```python
from build123d import *

# Parameters (mm, degrees)
SKETCH_1_W          = 88
SKETCH_1_H          = 60.2
EXTRUDE_1_DEPTH     = 16
SKETCH_1_4_R        = 5
SKETCH_1_4_R_2      = 9.5
EXTRUDE_3_DEPTH     = 23
SKETCH_2_R          = 4
EXTRUDE_4_DEPTH     = 30
CUT_EXTRUDE_3_DEPTH = 15
SKETCH_4_R          = 1.5
CUT_EXTRUDE_4_DEPTH = 10
EXTRUDE_6_DEPTH     = 16
EXTRUDE_7_DEPTH     = 2
SKETCH_7_R          = 22.25
EXTRUDE_8_DEPTH     = 66.5


with BuildPart() as part:
    # 草图1 → 凸台-拉伸1 (new body)
    with BuildSketch(Plane(origin=(0, 0, 0), x_dir=(1, 0, 0), z_dir=(0, 1, 0))):
        Rectangle(SKETCH_1_W, SKETCH_1_H)
    extrude(amount=EXTRUDE_1_DEPTH)

    # 草图1<4> → 凸台-拉伸3 (add)
    with BuildSketch(Plane(origin=(0, 0, 0), x_dir=(1, 0, 0), z_dir=(0, 1, 0))):
        with Locations((-20.4, 20)):
            Circle(SKETCH_1_4_R)
        with Locations((19.6, 20)):
            Circle(SKETCH_1_4_R)
        with Locations((19.6, -20)):
            Circle(SKETCH_1_4_R)
        with Locations((-20.4, -20)):
            Circle(SKETCH_1_4_R)
        with Locations((-20.4, 0)):
            Circle(SKETCH_1_4_R_2)
    extrude(amount=EXTRUDE_3_DEPTH)

    # 草图2 → 凸台-拉伸4 (add)
    with BuildSketch(Plane(origin=(0, 23, 0), x_dir=(1, 0, 0), z_dir=(0, 1, 0))):
        with Locations((-20.4, 0)):
            Circle(SKETCH_2_R)
    extrude(amount=EXTRUDE_4_DEPTH)

    # 草图3 → 切除-拉伸3 (cut)
    with BuildSketch(Plane(origin=(0, 53, 0), x_dir=(1, 0, 0), z_dir=(0, 1, 0))):
        with BuildLine():
            Line((-23.864101615, 2), (-16.935898385, 2))
            ThreePointArc((-16.935898385, 2), (-20.4, 4), (-23.864101615, 2))
        make_face()
    extrude(amount=-CUT_EXTRUDE_3_DEPTH, mode=Mode.SUBTRACT)

    # 草图4 → 切除-拉伸4 (cut)
    with BuildSketch(Plane(origin=(0, 23, 0), x_dir=(1, 0, 0), z_dir=(0, 1, 0))):
        with Locations((-20.4, 20)):
            Circle(SKETCH_4_R)
        with Locations((19.6, 20)):
            Circle(SKETCH_4_R)
        with Locations((19.6, -20)):
            Circle(SKETCH_4_R)
        with Locations((-20.4, -20)):
            Circle(SKETCH_4_R)
    extrude(amount=-CUT_EXTRUDE_4_DEPTH, mode=Mode.SUBTRACT)

    # 草图5 → 凸台-拉伸6 (add)
    with BuildSketch(Plane(origin=(0, 0, 0), x_dir=(1, 0, 0), z_dir=(0, 1, 0))):
        with BuildLine():
            Line((44, -30.1), (44, 30.1))
            ThreePointArc((44, 30.1), (50.801977879, 0), (44, -30.1))
        make_face()
    extrude(amount=EXTRUDE_6_DEPTH)

    # 草图6 → 凸台-拉伸7 (add)
    with BuildSketch(Plane.XZ):
        with BuildLine():
            Line((18, -16), (48.948878029, -16))
            ThreePointArc((48.948878029, -16), (50.801977879, 0), (48.948878029, 16))
            Line((48.948878029, 16), (18, 16))
            Line((18, 16), (18, -16))
        make_face()
    extrude(amount=EXTRUDE_7_DEPTH)

    # 草图7 → 凸台-拉伸8 (add)
    with BuildSketch(Plane.XZ.offset(2)):
        with Locations((34.40098894, 0)):
            Circle(SKETCH_7_R)
    extrude(amount=EXTRUDE_8_DEPTH)


solid = part.part
```
Could you check a few things on this model? Use its own coordinates, in mm. A direction names the side the tool comes from. Give positions to 0.01 mm unless a question says otherwise; leave off trailing zeros. Order: outer loops, then holes, each group sorted by start corner. A loop starts at its lowest first (then second) coordinate and runs counter-clockwise, first axis right, second up.
Q1. If I drill on line 1 along X through (y, z) = (21, -20); line 2 along Z through (x, y) = (19.6, 19); line 3 along Z through (x, y) = (19, 15), over which ranges is the centre line in solid material (lowest first)?
Q2. Suppose I cut it at B-B, the plane z = 20. Write out the boundary of the cut face in (x, y), and give its area (3 significant figures).
Q3. We'd pull the mould along Z, two halves only. Please class faces 1 (the flat face through (34, -68.5, 0)), 2 (the cylindrical face through (18.1, 18.07, 19.93)), 3 (the flat face through (-1, 8, 30.1)): +Z half, -Z half, draft (parallel to the pull), parting line (faces both ways), or undercut.
Q4. Suppose I cut it at A-A, the plane z = 0. Write out the boundary of the cut face in (x, y), and give its area (3 significant figures).
Q5. I'm going to push flat-ended pins straight in: P1, Ø1, axis at x = -21, z = -3, coming from the +Y side; P2, Ø2, axis at y = -6, z = -15.5, coming from the +X side; P3, Ø11, axis at x = 19, z = -22, coming from the +Y side; P4, Ø9.5, axis at x = -21.5, z = -4.5, coming from the +Y side. Where does each tip first touch, or does it pass through?
Q6. For faces 4 (the flat face through (-22, 23, 21)), 5 (the flat face through (-20, 46, -2)), 6 (the flat face through (-16, 23, 0)), which set-ups out of +Z, -Z, +X, -X, +Y, -Y let a thin tool reach every point of the face, with its end or its side?
Q7. Suppose I cut it at D-D, the plane y = 41. Write out the boundary of the cut face in (x, z).
Solution:
1. line 1: x = -25.4 to -21.9, -18.9 to -15.4, 14.6 to 18.1, 21.1 to 24.6
1. line 2: z = -25 to -21.5, -18.5 to -15, 15 to 18.5, 21.5 to 25
1. line 3: z = -30.1 to -21.37, -18.63 to 18.63, 21.37 to 30.1
2. outline: (-44, 0) - (47.88, 0) - (47.88, 16) - (24.6, 16) - (24.6, 23) - (21.1, 23) - (21.1, 13) - (18.1, 13) - (18.1, 23) - (14.6, 23) - (14.6, 16) - (-15.4, 16) - (-15.4, 23) - (-18.9, 23) - (-18.9, 13) - (-21.9, 13) - (-21.9, 23) - (-25.4, 23) - (-25.4, 16) - (-44, 16) - close; (24.65, -68.5) - (44.15, -68.5) - (44.15, -2) - (24.65, -2) - close
2. area: 2,850 mm2
3. face 1: draft
3. face 2: undercut
3. face 3: +Z half
4. outline: (-44, 0) - (18, 0) - (18, -2) - (12.15, -2) - (12.15, -68.5) - (56.65, -68.5) - (56.65, -2) - (50.8, -2) - (50.8, 16) - (-10.9, 16) - (-10.9, 23) - (-16.4, 23) - (-16.4, 53) - (-24.4, 53) - (-24.4, 23) - (-29.9, 23) - (-29.9, 16) - (-44, 16) - close
4. area: 4,910 mm2
5. P1: stops at y = 38
5. P2: stops at x = 51.28
5. P3: stops at y = 23
5. P4: stops at y = 53
6. face 4: +Z, +X, -X, +Y
6. face 5: -Z, +X, -X, +Y
6. face 6: +Y
7. outline: (-23.86, -2) - (-16.94, -2) arc R4 ccw (long way) to start
